Design review of the part built by this model. Coordinates are the model's own, in mm. A direction names the side the tool comes from. Round coordinates to 2 decimals unless told otherwise and drop trailing zeros. Write each loop counter-clockwise with the first axis right and the second up, starting at its lowest first coordinate (ties: lowest second). Pieces come first, ordered by that corner, then holes. Notation, with made-up numbers: (53.25, 10.5) -> (105.25, 10.5) arc R16 cw to (105.25, 34.5) -> close; hole circle Ø9 at (75.25, 16). An arc over 180 degrees is marked (long way). Write item = value, one per line. Start each with the question number.
Item 1: Machinability: for faces 1 (the cylindrical face through (98.52, 32.9, 0.09)), 2 (the flat face through (-1.4, -22.4, 10.1)), 3 (the flat face through (-1, -30, 0)), which of the approach directions +Z, -Z, +X, -X, +Y, -Y give a long, thin tool a straight path to every point of the face, cutting with its end or side? Answer none if there is none.
Item 2: Add section B-B, the plane x = -82. State the section outline as (y, z) points.
Item 3: Add section A-A, the plane z = -12. State the section outline as (x, y) points, then the cut area to 3 significant figures.
Item 4: Mouldability with a two-part tool opening along Z and no side actions: class faces 4 (the flat face through (-1, 18, 17.5)), 5 (the flat face through (100, -1, 4)), 6 (the flat face through (-1.4, -22.4, -10.1)), 7 (the flat face through (97, -5.1, 2.3)) as released by +Z, released by -Z, zero draft, split by the parting line, or undercut.
Item 5: Add section C-C, the plane z = 7. State the section outline as (x, y) points.
Item 6: To check wall thickness, follow L1, parallel to X at y = -22, z = 11; L2, parallel to Y at x = -84, z = 2; L3, parallel to Y at x = -7, z = 12. State the ranges of each line that lie inside material, in increasing order.
Item 7: For pin 1 Ø1.5 at (x, y) = (98, 35.5) entering from +Z; pin 2 Ø5.5 at (x, z) = (7, 0) entering from -Y, all flat-tipped, find the tip position at first contact; note any pin that passes through.
from build123d import *

# Parameters (mm, degrees)
F1_DEPTH      = 17.5
F1_DEPTH_BACK = 17.5
F2_SIZE       = 15
F3_SIZE       = 7.5
F4_R          = 2.1
F5_DEPTH      = 3
F7_DEPTH      = 0.01


with BuildPart() as f1:
    # F0 (on Top) → F1 (new body, two sides)
    with BuildSketch(Plane.XY) as f1_sk:
        Polygon((100, -50), (100, 50), (-100, 50), (-100, -50), (-97, -50), (-97, -30), (97, -30), (97, -50), align=None)
    extrude(amount=F1_DEPTH)
    extrude(f1_sk.sketch, amount=-F1_DEPTH_BACK)

    # F2
    f2_edges = [f1.edges().sort_by_distance(p)[0] for p in [
        (0, -30, 17.5),
        (0, -30, -17.5),
    ]]
    chamfer(f2_edges, length=F2_SIZE)

    # F3
    f3_edges = [f1.edges().sort_by_distance(p)[0] for p in [
        (98.5, -50, 17.5),
        (98.5, -50, -17.5),
        (-98.5, -50, 17.5),
        (-98.5, -50, -17.5),
    ]]
    chamfer(f3_edges, length=F3_SIZE)

    # F4 (on face) → F5 (cut)
    with BuildSketch(Plane.YZ.offset(100)):
        with BuildLine():
            ThreePointArc((42.5, 0), (41.767767, 1.767767), (40, 2.5))
            Line((40, 2.5), (30, 2.5))
            ThreePointArc((30, 2.5), (28.232233, 1.767767), (27.5, 0))
            ThreePointArc((27.5, 0), (28.232233, -1.767767), (30, -2.5))
            Line((30, -2.5), (40, -2.5))
            ThreePointArc((40, -2.5), (41.767767, -1.767767), (42.5, 0))
        make_face()
        with Locations((35, 0)):
            Circle(F4_R, mode=Mode.SUBTRACT)
        with BuildLine():
            ThreePointArc((2.5, 0), (1.767767, 1.767767), (0, 2.5))
            Line((0, 2.5), (-10, 2.5))
            ThreePointArc((-10, 2.5), (-11.767767, 1.767767), (-12.5, 0))
            ThreePointArc((-12.5, 0), (-11.767767, -1.767767), (-10, -2.5))
            Line((-10, -2.5), (0, -2.5))
            ThreePointArc((0, -2.5), (1.767767, -1.767767), (2.5, 0))
        make_face()
        with Locations((-5, 0)):
            Circle(F4_R, mode=Mode.SUBTRACT)
    extrude(amount=-F5_DEPTH, mode=Mode.SUBTRACT)

    # F6 (on face) → F7 (cut)
    with BuildSketch(Plane.XY.offset(17.5)):
        Polygon((100, 50), (97, 50), (97, -15), (97, -42.5), (100, -42.5), align=None)
        Polygon((-97, 50), (-100, 50), (-100, -42.5), (-97, -42.5), (-97, -15), align=None)
    extrude(amount=-F7_DEPTH, mode=Mode.SUBTRACT)


solid = f1.part
Result set:
q1.face_1 = +X
q1.face_2 = +Z, -Y
q1.face_3 = +Z, -Z, -Y
q2.outline = (-30, -2.5) -> (-15, -17.5) -> (50, -17.5) -> (50, 17.5) -> (-15, 17.5) -> (-30, 2.5) -> close
q3.outline = (-100, -48) -> (-97, -48) -> (-97, -20.5) -> (97, -20.5) -> (97, -48) -> (100, -48) -> (100, 50) -> (-100, 50) -> close
q3.area = 14,300 mm²
q4.face_4 = released by +Z
q4.face_5 = zero draft
q4.face_6 = released by -Z
q4.face_7 = undercut
q5.outline = (-100, -50) -> (-97, -50) -> (-97, -25.5) -> (97, -25.5) -> (97, -50) -> (100, -50) -> (100, 50) -> (-100, 50) -> close
q6.L1 = -100 to -97, 97 to 100
q6.L2 = -30 to 50
q6.L3 = -20.5 to 50
q7.pin_1 = 17.49
q7.pin_2 = -30
